from build123d import *

# Parameters (mm, degrees)
SKETCH_1_W          = 30
SKETCH_1_H          = 10
SKETCH_1_R          = 2.5
EXTRUDE_1_DEPTH     = 10
CUT_EXTRUDE_1_REACH = 34.016
SKETCH_2_R          = 4.5


with BuildPart() as part:
    # 草圖1 → 填料-伸長1 (new body)
    with BuildSketch(Plane.XY):
        Rectangle(SKETCH_1_W, SKETCH_1_H)
        with Locations((-10, 0)):
            Circle(SKETCH_1_R, mode=Mode.SUBTRACT)
        with Locations((5, 0)):
            Circle(SKETCH_1_R, mode=Mode.SUBTRACT)
    extrude(amount=EXTRUDE_1_DEPTH)

    # 草圖2 → 除料-伸長1 (cut, up to next)
    with BuildSketch(Plane(origin=(15, 0, 0), x_dir=(0, 0, -1), z_dir=(1, 0, 0)), mode=Mode.PRIVATE) as cut_extrude_1_sk1:
        with Locations((-5, 7.25)):
            Circle(SKETCH_2_R)
    cut_extrude_1_tool1 = extrude(cut_extrude_1_sk1.sketch, amount=-CUT_EXTRUDE_1_REACH, mode=Mode.PRIVATE) & part.part
    add(cut_extrude_1_tool1.solids().sort_by_distance((15, 7.25, 5))[0], mode=Mode.SUBTRACT)


solid = part.part
Work out the finished part from the listing and answer in its coordinate system (mm). Give positions to 0.01 mm unless a question says otherwise; leave off trailing zeros. Loops run counter-clockwise (first coordinate to the right, second up) from the corner with the lowest first, then second, coordinate; pieces in that order, holes last. Notation, with made-up numbers: M 19,35.5 L 39,35.5 A3 cw 39,39.5 Z; hole C 40.25,-24.75 d6. An arc over 180 degrees is marked long. Use CSV: the item, a comma, the result in double quotes.
1) Determine the mould class of faces 1 (the cylindrical face through (7.385, 0.751, 4.93)), 2 (the flat face through (0, 0, 10)), 3 (the flat face through (-15, -1, 5)), 4 (the flat face through (15, -1, 5)) for opening direction X: released by +X, released by -X, zero draft, split by the parting line, or undercut.
Answer:
face 1,"undercut"
face 2,"zero draft"
face 3,"released by -X"
face 4,"released by +X"
2) Find section D-D on x = -5.25. Write down the section's boundary in (y, z), plus the area to 3 significant figures.
Answer:
outline,"M -5,0 L 5,0 L 5,1.1 A4.5 cw 5,8.9 L 5,10 L -5,10 Z"
area,"87.6 mm^2"
3) Find section B-B on x = 3.5. Write down the section's boundary in (y, z), plus the area to 3 significant figures.
Answer:
outline,"M -5,0 L -2,0 L -2,10 L -5,10 Z; M 2,0 L 5,0 L 5,1.1 A4.5 cw 5,8.9 L 5,10 L 2,10 Z"
area,"47.6 mm^2"
4) Given P1, Ø3, axis at x = -10, y = 0, coming from the -Z side, flat-ended and moving along its own axis, determine where the tip first touches the part or whether it passes through.
Answer:
P1,"through"
5) Find section C-C on y = 3.5. Write down the section's boundary in (x, z).
Answer:
outline,"M -15,0 L 15,0 L 15,2.51 L -15,2.51 Z; M -15,7.49 L 15,7.49 L 15,10 L -15,10 Z"
6) Find section A-A on y = -1.5. Write down the section's boundary in (x, z), plus the area to 3 significant figures.
Answer:
outline,"M -15,0 L -12,0 L -12,10 L -15,10 Z; M -8,0 L 3,0 L 3,10 L -8,10 Z; M 7,0 L 15,0 L 15,10 L 7,10 Z"
area,"220 mm^2"
7) Consider L1, parallel to X at y = -1.5, z = 2.25; L2, parallel to Y at x = -10, z = 5; L3, parallel to X at y = 2.25, z = 9.25. Determine where each line is inside the solid, lowest interval first.
Answer:
L1,"-15 to -12, -8 to 3, 7 to 15"
L2,"-5 to -2.5, 2.5 to 2.75"
L3,"-15 to -11.09, -8.91 to 3.91, 6.09 to 15"
